```python
from build123d import *

# Parameters (mm, degrees)
SKETCH2_W             = 39.3827
SKETCH2_H             = 7.62
BOSS_EXTRUDE2_DEPTH   = 4.064
BOSS_EXTRUDE2_2_DEPTH = 4.064
SKETCH2_3_W           = 39.3827
SKETCH2_3_H           = 60.96
SKETCH2_3_R           = 2.794
BOSS_EXTRUDE3_DEPTH   = 2.54


with BuildPart() as part:
    # Sketch2 → Boss-Extrude2 (new body)
    with BuildSketch(Plane(origin=(0, 0, 0), x_dir=(1, 0, 0), z_dir=(0, 1, 0))):
        with Locations((19.69135, 3.81)):
            Rectangle(SKETCH2_W, SKETCH2_H)
    extrude(amount=BOSS_EXTRUDE2_DEPTH)



with BuildPart() as body_2:
    # Sketch2 → Boss-Extrude2 2 (new body)
    with BuildSketch(Plane(origin=(0, 0, 0), x_dir=(1, 0, 0), z_dir=(0, 1, 0))):
        with Locations((19.69135, 72.39)):
            Rectangle(SKETCH2_W, SKETCH2_H)
    extrude(amount=BOSS_EXTRUDE2_2_DEPTH)


with BuildPart() as part_1:
    add(part.part)

    add(body_2.part)  # Boss-Extrude3 merges body 2
    # Sketch2_3 → Boss-Extrude3 (add)
    with BuildSketch(Plane(origin=(0, 0, 0), x_dir=(1, 0, 0), z_dir=(0, 1, 0))):
        with Locations((19.69135, 38.1)):
            Rectangle(SKETCH2_3_W, SKETCH2_3_H)
        Polygon((12.954, 63.5), (12.954, 38.1), (12.954, 12.7), (5.08, 12.7), (5.08, 63.5), align=None, mode=Mode.SUBTRACT)
        with Locations(Location((23.971932262, 22.733, 0), (0, 0, 270))):
            Circle(SKETCH2_3_R, mode=Mode.SUBTRACT)
        with Locations(Location((23.971932262, 53.467, 0), (0, 0, 270))):
            Circle(SKETCH2_3_R, mode=Mode.SUBTRACT)
    extrude(amount=BOSS_EXTRUDE3_DEPTH)


solid = part_1.part
```
Geometry check sheet. Reference: the model listing, model coordinates, mm. A direction names the side the tool comes from. Coordinates: 2 decimals unless noted, no trailing zeros. Order: outer loops, then holes, each group sorted by start corner. A loop starts at its lowest first (then second) coordinate and runs counter-clockwise, first axis right, second up. Notation, with made-up numbers: (22, -26.75) - (59, -26.75) arc R12 cw to (59, -6.75) - close; hole circle Ø1 at (-20.5, -6). An arc over 180 degrees is marked (long way). Answer as a JSON object with one key per item and string values. Group by question number.
Item 1: Scan lines: probe 1 along X at (y, z) = (0.5, -23); probe 2 along Z at (x, y) = (24, 1.55); probe 3 along X at (y, z) = (0.55, -41.5). Record each from-to range of solid material in increasing order.
Item 2: Depth check by flat-ended pin: pin 1 Ø19.5 at (x, z) = (23, -24.5) entering from +Y. Enter the tip coordinate at first touch or a pass-through.
Item 3: Sectioned sample at D-D, the plane z = -55. Record the cut outline in (x, y), and give its area (3 significant figures).
Item 4: Tool access check on faces 4 (the face through (19, 3, -68.58)), 5 (the face through (0, 2, -38)), 6 (the face through (9, 1, -63.5)). Record the directions out of +Z, -Z, +X, -X, +Y, -Y that give a thin tool (end or side, any length) a straight path to the whole face; none if there is none.
Item 5: Draft check along Z on faces 1 (the face through (19, 4.064, -4)), 2 (the face through (19, 2, 0)), 3 (the face through (5.08, 1, -38)). Enter one of: +Z half, -Z half, draft (parallel to the pull), parting line (faces both ways), or undercut.
Item 6: Sectioned sample at A-A, the plane y = 3.4. Record the cut outline in (x, z), and give its area (3 significant figures).
Item 7: Sectioned sample at C-C, the plane x = 9.5. Record the cut outline in (y, z), and give its area (3 significant figures).
Item 8: Sectioned sample at B-B, the plane z = -39. Record the cut outline in (x, y).
Resolved:
{
 "1": {"probe 1": "0 to 5.08, 12.95 to 21.19, 26.75 to 39.38", "probe 2": "-76.2 to -56.26, -50.67 to -25.53, -19.94 to 0", "probe 3": "0 to 5.08, 12.95 to 39.38"},
 "2": {"pin 1": "y = 2.54"},
 "3": {"outline": "(0, 0) - (5.08, 0) - (5.08, 2.54) - (0, 2.54) - close; (12.95, 0) - (21.64, 0) - (21.64, 2.54) - (12.95, 2.54) - close; (26.31, 0) - (39.38, 0) - (39.38, 2.54) - (26.31, 2.54) - close", "area": "68.2 mm^2"},
 "4": {"face 4": "+X, -X, +Y", "face 5": "+Z, -Z, -X, +Y, -Y", "face 6": "+Y, -Y"},
 "5": {"face 1": "draft", "face 2": "+Z half", "face 3": "undercut"},
 "6": {"outline": "(0, -76.2) - (39.38, -76.2) - (39.38, -68.58) - (0, -68.58) - close; (0, -7.62) - (39.38, -7.62) - (39.38, 0) - (0, 0) - close", "area": "600 mm^2"},
 "7": {"outline": "(0, -76.2) - (4.06, -76.2) - (4.06, -68.58) - (2.54, -68.58) - (2.54, -63.5) - (0, -63.5) - close; (0, -12.7) - (2.54, -12.7) - (2.54, -7.62) - (4.06, -7.62) - (4.06, 0) - (0, 0) - close", "area": "87.7 mm^2"},
 "8": {"outline": "(0, 0) - (5.08, 0) - (5.08, 2.54) - (0, 2.54) - close; (12.95, 0) - (39.38, 0) - (39.38, 2.54) - (12.95, 2.54) - close"}
}
